```python
from build123d import *

# Parameters (mm, degrees)
SKETCH1_R           = 15
BOSS_EXTRUDE1_DEPTH = 100


with BuildPart() as part:
    # Sketch1 → Boss-Extrude1 (new body)
    with BuildSketch(Plane.XY):
        with BuildLine():
            Line((70.134297521, 0), (-84.865702479, 0))
            Line((-84.865702479, 0), (-84.865702479, 106))
            ThreePointArc((-84.865702479, 106), (-83.694129604, 108.828427125), (-80.865702479, 110))
            Line((-80.865702479, 110), (-28.865702479, 110))
            ThreePointArc((-28.865702479, 110), (-26.037275355, 108.828427125), (-24.865702479, 106))
            Line((-24.865702479, 106), (-24.865702479, 83.851648071))
            ThreePointArc((-24.865702479, 83.851648071), (-23.797014915, 81.129992802), (-21.161998776, 79.862637103))
            ThreePointArc((-21.161998776, 79.862637103), (10.48963658, 65.355339059), (24.996934624, 33.703703704))
            ThreePointArc((24.996934624, 33.703703704), (26.264290322, 31.068687565), (28.985945592, 30))
            Line((28.985945592, 30), (66.134297521, 30))
            ThreePointArc((66.134297521, 30), (68.962724645, 28.828427125), (70.134297521, 26))
            Line((70.134297521, 26), (70.134297521, 0))
        make_face()
        with Locations(Location((-54.865702479, 80, 0), (0, 0, 180))):
            Circle(SKETCH1_R, mode=Mode.SUBTRACT)
        with BuildLine():
            Line((0.824762678, 30), (-60.865702479, 30))
            ThreePointArc((-60.865702479, 30), (-63.694129604, 31.171572875), (-64.865702479, 34))
            Line((-64.865702479, 34), (-64.865702479, 56))
            ThreePointArc((-64.865702479, 56), (-63.694129604, 58.828427125), (-60.865702479, 60))
            Line((-60.865702479, 60), (-24.865702479, 60))
            ThreePointArc((-24.865702479, 60), (-5.352393412, 52.786635759), (4.777141933, 34.615384615))
            ThreePointArc((4.777141933, 34.615384615), (3.862980779, 31.398225458), (0.824762678, 30))
        make_face(mode=Mode.SUBTRACT)
    extrude(amount=BOSS_EXTRUDE1_DEPTH)


solid = part.part
```
Verification items for the finished model (mm, model axes). A direction names the side the tool comes from. Coordinates: 2 decimals unless noted, no trailing zeros. Order: outer loops, then holes, each group sorted by start corner. A loop starts at its lowest first (then second) coordinate and runs counter-clockwise, first axis right, second up. Notation, with made-up numbers: (70.5, 56.5) -> (120.5, 56.5) arc R25 ccw to (120.5, 68.5) -> close; hole circle Ø8 at (67.25, -8). An arc over 180 degrees is marked (long way). Answer as CSV lines item,"result". Start each with the question number.
1) Material ranges on L1, parallel to Y at x = -35, z = 86; L2, parallel to Y at x = -56, z = 67.5; L3, parallel to Y at x = -63, z = 77, recorded low to high. Write a range as [from, to].
2) Cross-section at D-D, the plane x = 56.5. Record the boundary of the cut face in (y, z), then the cut area to 3 significant figures.
3) Cross-section at C-C, the plane y = 51. Record the boundary of the cut face in (x, z).
4) Release check for a two-part mould opening along Y. For faces 1 (the face through (70.134, 13, 49)), 2 (the face through (-63.725, 58.797, 49.3)), 3 (the face through (10.136, 65.706, 49.3)), 4 (the face through (-64.866, 45, 49)) record: released by +Y, released by -Y, zero draft, split by the parting line, or undercut.
5) Gauge pin test, flat ends, axial feed: pin 1 Ø12 at (x, z) = (-0.5, 67.5) entering from -Y; pin 2 Ø3 at (x, z) = (49, 27.5) entering from +Y; pin 3 Ø12 at (x, z) = (22.5, 53.5) entering from +Y; pin 4 Ø6.5 at (y, z) = (99, 39.5) entering from +X. Record the tip position at first contact, or that the pin passes through.
6) Cross-section at A-A, the plane x = -38. Record the boundary of the cut face in (y, z), then the cut area to 3 significant figures.
7) Cross-section at B-B, the plane z = 82. Record the boundary of the cut face in (x, y), then the cut area to 3 significant figures.
8) Set-up check for faces 5 (the face through (-43, 60, 49)), 6 (the face through (-24.866, 95, 49)), 7 (the face through (-83.725, 108.797, 49.3)): record each of +Z, -Z, +X, -X, +Y, -Y from which the full face is reachable in a straight line by a thin tool's end or side.
Conclusion:
1,L1,"y = [0, 30], [60, 110]"
1,L2,"y = [0, 30], [60, 65.04], [94.96, 110]"
1,L3,"y = [0, 30.62], [59.38, 67.4], [92.6, 110]"
2,outline,"(0, 0) -> (30, 0) -> (30, 100) -> (0, 100) -> close"
2,area,"3,000 mm²"
3,outline,"(-84.87, 0) -> (-64.87, 0) -> (-64.87, 100) -> (-84.87, 100) -> close; (-3.44, 0) -> (20.51, 0) -> (20.51, 100) -> (-3.44, 100) -> close"
4,face 1,"zero draft"
4,face 2,"undercut"
4,face 3,"released by +Y"
4,face 4,"undercut"
5,pin 1,"stops at y = 0"
5,pin 2,"stops at y = 30"
5,pin 3,"stops at y = 58.09"
5,pin 4,"stops at x = -24.87"
6,outline,"(0, 0) -> (30, 0) -> (30, 100) -> (0, 100) -> close; (60, 0) -> (110, 0) -> (110, 100) -> (60, 100) -> close"
6,area,"8,000 mm²"
7,outline,"(-84.87, 0) -> (70.13, 0) -> (70.13, 26) arc R4 ccw to (66.13, 30) -> (28.99, 30) arc R4 cw to (25, 33.7) arc R50 ccw to (-21.16, 79.86) arc R4 cw to (-24.87, 83.85) -> (-24.87, 106) arc R4 ccw to (-28.87, 110) -> (-80.87, 110) arc R4 ccw to (-84.87, 106) -> close; hole circle Ø30 at (-54.87, 80); hole (-64.87, 34) arc R4 ccw to (-60.87, 30) -> (0.82, 30) arc R4 ccw to (4.78, 34.62) arc R30 ccw to (-24.87, 60) -> (-60.87, 60) arc R4 ccw to (-64.87, 56) -> close"
7,area,"8,810 mm²"
8,face 5,"+Z, -Z"
8,face 6,"+Z, -Z, +X, +Y"
8,face 7,"+Z, -Z, -X, +Y"
